Autodesk Inventor part; units mm, degrees
ref_plane "YZ Plane" through (0, 0, 0) normal (1, 0, 0) x (0, 1, 0)
ref_plane "XZ Plane" through (0, 0, 0) normal (0, 1, 0) x (-1, 0, 0)
ref_plane "XY Plane" through (0, 0, 0) normal (0, 0, 1) x (1, 0, 0)
sketch "草图1" plane through (0, 0, 0) normal (0, 0, 1) x (1, 0, 0)
  circle A0 centre (0, 0) radius 2
  line L0 (1.7321, -3) -> (-1.7321, -3)
  line L1 (-1.7321, -3) -> (-3.4641, 0)
  line L2 (-3.4641, 0) -> (-1.7321, 3)
  line L3 (-1.7321, 3) -> (1.7321, 3)
  line L4 (1.7321, 3) -> (3.4641, 0)
  line L5 (3.4641, 0) -> (1.7321, -3)
  line L6 (0, 0) -> (0, 1.0765)
  point P0 (0, 3)
  dimension "d0" = 4
  dimension "d1" = 1.0765
  dimension "d2" = 6
extrude "拉伸1" add sketch "草图1" along normal blind 4
sketch "草图2" plane through (0, 0, 4) normal (0, 0, 1) x (1, 0, 0)
  circle A0 centre (0, 0) radius 4
  circle A1 centre (0, 0) radius 2
  dimension "d5" = 8
  dimension "d6" = 4
extrude "拉伸2" add sketch "草图2" along normal blind 1
thread "螺纹1"
fillet "圆角1" radius 0.25 13 edges at (-4, 0, 4) (1.7321, 3, 2) (2.5981, 1.5, 0) (0, 3, 0) (-2.5981, 1.5, 0) (-2.5981, -1.5, 0) (0, -3, 0) (2.5981, -1.5, 0) (1.7321, -3, 2) (3.4641, 0, 2) (-1.7321, -3, 2) (-3.4641, 0, 2) (-1.7321, 3, 2)
chamfer "倒角1" distance 0.25 angle 45 1 edges at (-2, 0, 0)
properties part number "刀轴端盖螺帽"
For this review, take the finished solid that the model builds, in its own axes (mm). A direction names the side the tool comes from. Give positions to 0.01 mm unless a question says otherwise; leave off trailing zeros. Loops run counter-clockwise (first coordinate to the right, second up) from the corner with the lowest first, then second, coordinate; pieces in that order, holes last.
Item 1: Take a section at D-D, the plane z = 4.1. State the section outline as (x, y) points.
Item 2: Take a section at C-C, the plane z = 4.75. State the section outline as (x, y) points.
Item 3: Insertion check: pin 1 (2.5 mm diameter, centred on x = -0.5, z = 3, fed in from -Y); pin 2 (1.6 mm diameter, centred on x = 0, z = 2, fed in from +Y); pin 3 (1 mm diameter, centred on x = 0.5, y = 0, fed in from +Z); pin 4 (3 mm diameter, centred on y = 1.5, z = 3.5, fed in from -X). Each pin has a flat end and moves straight along its axis. Give the tip position at first contact, or say it passes through.
Item 4: Tool access review of faces 4 (the flat face through (2.6, 1.5, 2.1)), 5 (the flat face through (2.6, -1.5, 2.1)), 6 (the flat face through (-2.6, 1.5, 2.1)): name each direction out of +Z, -Z, +X, -X, +Y, -Y from which nothing blocks a thin tool from reaching the whole face with its end or side.
Item 5: For line 1 along Y through (x, z) = (0, 2.6); line 2 along Y through (x, z) = (0.5, 2.85); line 3 along X through (y, z) = (1.25, 2.65), list the stretches that pass through material, from the lowest coordinate up.
Item 6: Take a section at A-A, the plane x = 0. State the section outline as (y, z) points, and give its area (3 significant figures).
Item 7: Draft analysis for pull direction Y (two halves, no side actions). For faces 1 (the flat face through (0, 3, 2)), 2 (the cylindrical face through (0, 2, 3)), 3 (the flat face through (0, -3, 2)), state which applies: +Y half, -Y half, draft (parallel to the pull), parting line (faces both ways), or undercut.
Item 8: Take a section at B-B, the plane z = 1.7. State the section outline as (x, y) points (3 decimals), and give its area (3 significant figures).
Calculated:
1. outline: circle Ø7.9 at (0, 0); hole circle Ø4 at (0, 0)
2. outline: circle Ø8 at (0, 0); hole circle Ø4 at (0, 0)
3. pin 1: stops at y = -3.99
3. pin 2: stops at y = 3
3. pin 3: passes through
3. pin 4: stops at x = -4
4. face 4: -Z, +X, +Y
4. face 5: -Z, +X, -Y
4. face 6: -Z, -X, +Y
5. line 1: y = -3 to -2, 2 to 3
5. line 2: y = -3 to -1.94, 1.94 to 3
5. line 3: x = -2.74 to -1.56, 1.56 to 2.74
6. outline: (-4, 4.25) arc R0.25 ccw to (-3.75, 4) - (-3, 4) - (-3, 0.25) arc R0.25 ccw to (-2.75, 0) - (-2.25, 0) - (-2, 0.25) - (-2, 5) - (-4, 5) - close; (2, 0.25) - (2.25, 0) - (2.75, 0) arc R0.25 ccw to (3, 0.25) - (3, 4) - (3.75, 4) arc R0.25 ccw to (4, 4.25) - (4, 5) - (2, 5) - close
6. area: 11.9 mm2
7. face 1: +Y half
7. face 2: undercut
7. face 3: -Y half
8. outline: (-3.392, -0.125) - (-1.804, -2.875) arc R0.25 ccw to (-1.588, -3) - (1.588, -3) arc R0.25 ccw to (1.804, -2.875) - (3.392, -0.125) arc R0.25 ccw to (3.392, 0.125) - (1.804, 2.875) arc R0.25 ccw to (1.588, 3) - (-1.588, 3) arc R0.25 ccw to (-1.804, 2.875) - (-3.392, 0.125) arc R0.25 ccw to start; hole circle Ø4 at (0, 0)
8. area: 18.6 mm2
